Model file for the job. Use its own axes, mm. Coordinates: 2 decimals unless noted, no trailing zeros. Order: outer loops, then holes, each group sorted by start corner. A loop starts at its lowest first (then second) coordinate and runs counter-clockwise, first axis right, second up. Notation, with made-up numbers: (43.5, 43.5) -> (69.5, 43.5) arc R34 cw to (69.5, 81.5) -> close; hole circle Ø3 at (16.25, 28.5). An arc over 180 degrees is marked (long way). Return JSON: item names as keys, results as strings. Group by question number.
1) Flat gauge pins, fed straight in: pin 1 (1.6 mm diameter, centred on x = -109, z = 2, fed in from +Y); pin 2 (8 mm diameter, centred on x = 50, y = -86.6, fed in from -Z); pin 3 (0.9 mm diameter, centred on y = 52, z = 1, fed in from +X); pin 4 (0.9 mm diameter, centred on x = 121.5, z = 1, fed in from +Y). Where does each tip first touch, or does it go through?
2) Cut at B-B (x = 33). Write the cut outline in (y, z).
3) Probe line 1 (X direction, y = 53, z = 0.9); line 2 (X direction, y = -6.5, z = 2.05); line 3 (Y direction, x = -54, z = 2.15). List the from-to ranges inside material, lowest first.
4) Cut at C-C (z = 0.95). State how many separate pieces and enclosed holes the cut face has, and give its area (3 significant figures).
5) Cut at A-A (y = -16.5). Write the cut outline in (x, z).
Solid Edge part; units mm, degrees
sketch "Sketch1" plane through (0, 0, 0) normal (0, 0, 1) x (1, 0, 0)
  line L0 (0, 0) -> (-140, 0)
  line L1 (-140, 0) -> (-140, 140)
  line L2 (-140, 140) -> (0, 140)
  line L3 (0, 140) -> (0, 0)
  circle A0 centre (-50, 86.6025) radius 2.5
  dimension "D1" = 140
  dimension "D2" = 140
  dimension "D3" = 0
extrude "Ajout_matière_1" add sketch "Sketch1" along normal blind 3
sketch "Sketch2" plane through (-70, 70, 3) normal (0, 0, 1) x (1, 0, 0)
  line L0 (-70, -38.1818) -> (-40, -38.1818)
  line L1 (-40, -38.1818) -> (-40, 41.8182)
  line L2 (-40, 41.8182) -> (-70, 41.8182)
  line L3 (-70, 41.8182) -> (-70, -38.1818)
  dimension "D1" = 40
  dimension "D2" = 70
extrude "Cutout1" cut sketch "Sketch2" against normal through all
sketch "Sketch3" plane through (-70, 70, 3) normal (0, 0, 1) x (1, 0, 0)
  line L0 (70, 70) -> (-70, 70)
  line L1 (-70, 70) -> (-70, 50)
  arc A0 (-70, 50) -> (70, 70) centre (70, -430) cw
  dimension "D1" = 70
extrude "Cutout2" cut sketch "Sketch3" against normal through all
mirror "Mirror1" about plane through (0, 0, 0) normal (1, 0, 0) of "Ajout_matière_1", "Cutout1", "Cutout2"
mirror "Mirror2" about plane through (0, 0, 0) normal (0, -1, 0) of "Ajout_matière_1", "Cutout1", "Cutout2", "Mirror1"
sketch "Sketch4" plane through (0, 0, 3) normal (0, 0, 1) x (1, 0, 0)
  line L0 (-112, 44.2182) -> (-108, 44.2182)
  line L1 (-108, 44.2182) -> (-108, 58.2182)
  line L2 (-108, 58.2182) -> (-112, 58.2182)
  line L3 (-112, 58.2182) -> (-112, 44.2182)
  line L4 (-88, 58.2182) -> (-84, 58.2182)
  line L5 (-84, 58.2182) -> (-84, 54.6682)
  line L6 (-84, 54.6682) -> (-73, 54.6682)
  line L7 (-73, 54.6682) -> (-73, 47.7682)
  line L8 (-73, 47.7682) -> (-84, 47.7682)
  line L9 (-84, 47.7682) -> (-84, 44.2182)
  line L10 (-84, 44.2182) -> (-88, 44.2182)
  line L11 (-88, 44.2182) -> (-88, 58.2182)
  dimension "D1" = 112
  dimension "D2" = 108
  dimension "D3" = 88
  dimension "D4" = 73
  dimension "D5" = 88
  dimension "D6" = 84
  dimension "D7" = 84
extrude "Cutout9" cut sketch "Sketch4" against normal through all
mirror "Mirror3" about plane through (0, 0, 0) normal (1, 0, 0) of "Cutout9"
mirror "Mirror4" about plane through (0, 0, 0) normal (0, -1, 0) of "Cutout9", "Mirror3"
sketch "Sketch5" plane through (0, 0, 3) normal (0, 0, 1) x (0, 1, 0)
  line L0 (22.5, 137) -> (-22.5, 137)
  line L1 (-22.5, 137) -> (-22.5, 133)
  line L2 (-22.5, 133) -> (22.5, 133)
  line L3 (22.5, 133) -> (22.5, 137)
  dimension "D1" = 22.5
  dimension "D2" = 22.5
extrude "Cutout13" cut sketch "Sketch5" against normal through all
mirror "Mirror5" about plane through (0, 0, 0) normal (1, 0, 0) of "Cutout13"
sketch "Sketch6" plane through (0, 0, 3) normal (0, 0, 1) x (0, 1, 0)
  line L0 (124, 81) -> (120, 81)
  line L1 (120, 81) -> (120, -81)
  line L2 (120, -81) -> (124, -81)
  line L3 (124, -81) -> (124, 81)
  dimension "D1" = 124
  dimension "D2" = 124
extrude "Cutout15" cut sketch "Sketch6" against normal through all
mirror "Mirror6" about plane through (0, 0, 0) normal (0, -1, 0) of "Cutout15"
properties material "Acier S235"
Answers below:
{
 "1": {"pin 1": "stops at y = 128.15", "pin 2": "stops at z = 0", "pin 3": "stops at x = 108", "pin 4": "stops at y = 125.13"},
 "2": {"outline": "(-138.91, 0) -> (-124, 0) -> (-124, 3) -> (-138.91, 3) -> close; (-120, 0) -> (120, 0) -> (120, 3) -> (-120, 3) -> close; (124, 0) -> (138.91, 0) -> (138.91, 3) -> (124, 3) -> close"},
 "3": {"line 1": "x = -108 to -88, -73 to 73, 88 to 108", "line 2": "x = -140 to -137, -133 to 133, 137 to 140", "line 3": "y = -137.08 to -124, -120 to 120, 124 to 137.08"},
 "4": {"separate pieces": "1", "enclosed holes": "12", "area": "62,700 mm^2"},
 "5": {"outline": "(-140, 0) -> (-137, 0) -> (-137, 3) -> (-140, 3) -> close; (-133, 0) -> (133, 0) -> (133, 3) -> (-133, 3) -> close; (137, 0) -> (140, 0) -> (140, 3) -> (137, 3) -> close"}
}
